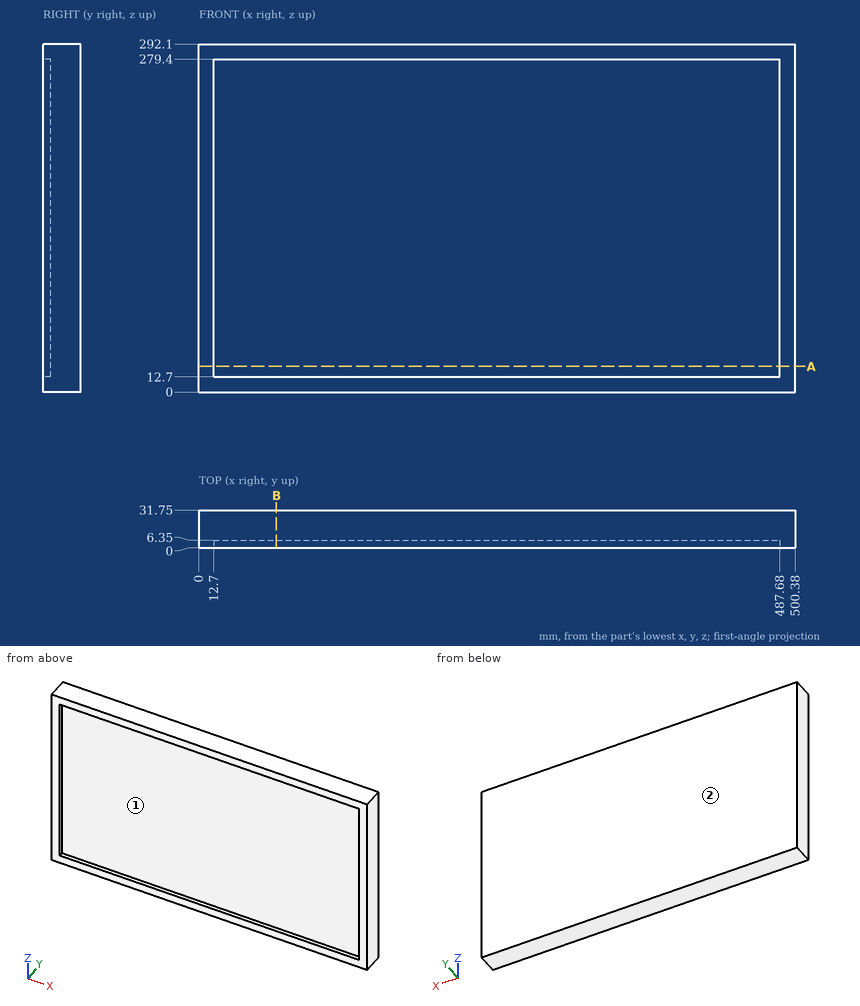
Design review of the part shown in the three views and the two pictorial views. Dimensions are in mm from the part's minimum x, y and z. Give positions to 0.01 mm unless a question says otherwise; leave off trailing zeros. Loops run counter-clockwise (first coordinate to the right, second up) from the corner with the lowest first, then second, coordinate; pieces in that order, holes last. Notation, with made-up numbers: M 57,-14.75 L 101,-14.75 A18 ccw 101,9.25 Z; hole C 33.5,-7 d5. An arc over 180 degrees is marked long. Answer as a JSON object with one key per item and string values. Group by question number.
Q1. Add section B-B on x = 65. Give the boundary of the cut face in (y, z).
Q2. Add section A-A on z = 21.5. Give the boundary of the cut face in (x, y).
Q3. Insertion check: P1, Ø5, axis at y = 20, z = 258.5, coming from the -X side; P2, Ø1.5, axis at x = 276, z = 52.5, coming from the -Y side. Each pin has a flat end and moves straight along its axis. Give the tip position at first contact, or say it passes through.
Q4. For probe 1 along Z at (x, y) = (325, 2); probe 2 along Y at (x, z) = (361.5, 274); probe 3 along X at (y, z) = (4, 170.5), list the stretches that pass through material, from the lowest coordinate up. Write a range as [from, to].
Q5. Mouldability with a two-part tool opening along X and no side actions: class the marked faces 1 and 2 as +X half, -X half, draft (parallel to the pull), parting line (faces both ways), or undercut.
Checked values:
{
 "1": {"outline": "M 0,0 L 31.75,0 L 31.75,292.1 L 0,292.1 L 0,279.4 L 6.35,279.4 L 6.35,12.7 L 0,12.7 Z"},
 "2": {"outline": "M 0,0 L 12.7,0 L 12.7,6.35 L 487.68,6.35 L 487.68,0 L 500.38,0 L 500.38,31.75 L 0,31.75 Z"},
 "3": {"P1": "x = 0", "P2": "y = 6.35"},
 "4": {"probe 1": "[0, 12.7], [279.4, 292.1]", "probe 2": "[6.35, 31.75]", "probe 3": "[0, 12.7], [487.68, 500.38]"},
 "5": {"face 1": "undercut", "face 2": "draft"}
}
